```python
from build123d import *

# Parameters (mm, degrees)
F1_DEPTH = 12.7
F2_W     = 12.7
F2_H     = 121.92
F3_DEPTH = 19.05


with BuildPart() as f1:
    # F0 (on Front) → F1 (new body)
    with BuildSketch(Plane.XZ):
        Polygon((0, 326.5288198487), (-320.0168273829, 0), (-189.0380174544, -89.7601038052), align=None)
    extrude(amount=F1_DEPTH)

    # F2 (on face) → F3 (join)
    with BuildSketch(Plane(origin=(-122.9286422393, 0, 55.8222558826), x_dir=(0, 1, 0), z_dir=(0.9105182057, 0, -0.4134689796))):
        with Locations((-6.35, 171.261092267)):
            Rectangle(F2_W, F2_H)
        with Locations((-6.35, -49.0228463048)):
            Rectangle(F2_W, F2_H)
    extrude(amount=F3_DEPTH)


solid = f1.part
```
Check sheet for the modelled part. Datum: model origin and axes. Units: mm. A direction names the side the tool comes from. Give positions to 0.01 mm unless a question says otherwise; leave off trailing zeros. Write each loop counter-clockwise with the first axis right and the second up, starting at its lowest first coordinate (ties: lowest second). Pieces come first, ordered by that corner, then holes. Notation, with made-up numbers: (78, -7) -> (83, -7) arc R11 ccw to (83, 3) -> close; hole circle Ø5 at (10, 13.25). An arc over 180 degrees is marked (long way). Use CSV: the item, a comma, the result in double quotes. Start each with the question number.
Q1. Cross-section at B-B on x = -113. Enter the section's corners in (y, z).
Q2. Cross-section at D-D on x = -67. Enter the section's corners in (y, z), and give its area (3 significant figures).
Q3. Scan lines: line 1 along Z through (x, y) = (-46, -10.5); line 2 along X through (y, z) = (-5, 28.5); line 3 along Z through (x, y) = (-18, -11.25). Record each from-to range of solid material in increasing order.
Q4. Depth check by flat-ended pin: P1, Ø2, axis at x = -54, z = 206, coming from the +Y side; P2, Ø1.5, axis at y = -4.5, z = 222, coming from the -X side; P3, Ø4, axis at y = -11, z = 218, coming from the -X side; P4, Ø1, axis at y = -10, z = 20, coming from the -X side. Enter the tip coordinate at first touch or a pass-through.
Q5. Cross-section at A-A on y = -7.5. Enter the section's corners in (x, z).
Q6. Cross-section at C-C on z = 71.5. Enter the section's corners in (x, y), and give its area (3 significant figures).
Q7. Release check for a two-part mould opening along X. For faces 1 (the flat face through (-68.77, -6.44, 152.37)), 2 (the flat face through (-161, -12.7, 73)), 3 (the flat face through (-18.4, -6.4, 263.4)), 4 (the flat face through (-159.852, -6.439, -48.202)) record: +X half, -X half, draft (parallel to the pull), parting line (faces both ways), or undercut.
Q8. Tool access check on faces 5 (the flat face through (-125.5, -6.44, 4.09)), 6 (the flat face through (-109.442, -6.439, 62.808)). Record the directions out of +Z, -Z, +X, -X, +Y, -Y that give a thin tool (end or side, any length) a straight path to the whole face; none if there is none.
Working result:
1,outline,"(-12.7, 31.61) -> (0, 31.61) -> (0, 64.42) -> (-12.7, 64.42) -> close; (-12.7, 77.69) -> (0, 77.69) -> (0, 211.23) -> (-12.7, 211.23) -> close"
2,outline,"(-12.7, 151.57) -> (0, 151.57) -> (0, 258.17) -> (-12.7, 258.17) -> close"
2,area,"1,350 mm^2"
3,line 1,"z = 179.16 to 279.59"
3,line 2,"x = -292.09 to -114.41"
3,line 3,"z = 240.82 to 263.22, 286.89 to 308.16"
4,P1,"stops at y = 0"
4,P2,"stops at x = -103.18"
4,P3,"stops at x = -108.32"
4,P4,"stops at x = -300.91"
5,outline,"(-320.02, 0) -> (-189.04, -89.76) -> (-168.4, -44.32) -> (-151.06, -52.2) -> (-100.65, 58.81) -> (-117.99, 66.69) -> (-77.32, 156.25) -> (-59.98, 148.38) -> (-9.57, 259.39) -> (-26.91, 267.26) -> (0, 326.53) -> close"
6,outline,"(-249.94, -12.7) -> (-115.81, -12.7) -> (-115.81, 0) -> (-249.94, 0) -> close"
6,area,"1,700 mm^2"
7,face 1,"undercut"
7,face 2,"draft"
7,face 3,"+X half"
7,face 4,"undercut"
8,face 5,"-Z, +X, +Y, -Y"
8,face 6,"+X, +Y, -Y"
